Input: part model. Units: mm. Frame: model coordinates. A direction names the side the tool comes from. Coordinates: 2 decimals unless noted, no trailing zeros.
1) Section query A-A (z = 2). State how many separate pieces and enclosed holes the cut face has, then the cut area to 3 significant figures.
2) Set-up query: faces 1 (the flat face through (132, -3.5, 3)), 2 (the cylindrical face through (36.819, -50.474, 4.521)), 3 (the flat face through (122.848, -37.563, 2.958)), 4 (the flat face through (-135, -1, 3)), 5 (the flat face through (-75, 83, 3)). Return all of +Z, -Z, +X, -X, +Y, -Y with unobstructed straight access to the full face (end or side cutting, diameter ignored); none if empty.
3) Draft query along Y for faces 6 (the flat face through (-35, 106.5, 3)), 7 (the flat face through (-72, 75.5, 3)), 8 (the flat face through (65, 109, 3)), 9 (the flat face through (110.085, -35.626, 2.958)). Return one class per face: pulls with the +Y half, pulls with the -Y half, needs draft (parallel to the pull), parting line crosses it, or undercut.
4) Pin query (flat end, axial travel): pin 1 Ø3 at (y, z) = (37, 2.5) entering from +X; pin 2 Ø5 at (x, y) = (132, 9) entering from +Z; pin 3 Ø2 at (y, z) = (-85, 3.5) entering from +X. Return the tip coordinate at first contact, or that it passes through.
5) Line query: L1, parallel to Y at x = 102.5, z = 3.75; L2, parallel to X at y = 97.5, z = 2.4; L3, parallel to Y at x = -101.5, z = 2. Output: solid intervals per line, ascending.
from build123d import *

# Parameters (mm, degrees)
ESQUISSE1_W                   = 270
ESQUISSE1_H                   = 213
BOSS_EXTRU_1_DEPTH            = 6
ESQUISSE3_R                   = 9.45
ESQUISSE3_R_2                 = 1.5
ENL_V_MAT_EXTRU_1_DEPTH       = 10
ENL_V_MAT_EXTRU_11_DEPTH      = 173.055950202
ENL_V_MAT_EXTRU_11_DEPTH_BACK = 173.055950202
ESQUISSE7_W                   = 6
ESQUISSE7_H                   = 30
ESQUISSE7_H_2                 = 27
ENL_V_MAT_EXTRU_13_DEPTH      = 10
ESQUISSE8_W                   = 40
ESQUISSE8_H                   = 6
BOSS_EXTRU_2_DEPTH            = 6
ENL_V_MAT_EXTRU_14_DEPTH      = 10
ENL_V_MAT_EXTRU_15_DEPTH      = 6
ESQUISSE11_W                  = 6
ESQUISSE11_H                  = 15
ENL_V_MAT_EXTRU_16_DEPTH      = 10
ESQUISSE14_W                  = 30
ESQUISSE14_H                  = 6
BOSS_EXTRU_3_DEPTH            = 6
ENL_V_MAT_EXTRU_18_DEPTH      = 176.833017377
ESQUISSE17_R                  = 2.995
ESQUISSE17_R_2                = 3
ENL_V_MAT_EXTRU_20_DEPTH      = 3
ESQUISSE18_R                  = 1.5
ENL_V_MAT_EXTRU_21_DEPTH      = 13


with BuildPart() as part:
    # Esquisse1 → Boss.-Extru.1 (new body)
    with BuildSketch(Plane.XY):
        Rectangle(ESQUISSE1_W, ESQUISSE1_H)
    extrude(amount=BOSS_EXTRU_1_DEPTH)

    # Esquisse3 → Enlèv. mat.-Extru.1 (cut)
    with BuildSketch(Plane.XY.offset(6)):
        with Locations((-100, -21.5)):
            Circle(ESQUISSE3_R)
        with Locations((35.99, -3.47)):
            Circle(ESQUISSE3_R_2)
        with Locations((43.49, 9.52)):
            Circle(ESQUISSE3_R_2)
        with Locations((44.65, -8.50726277)):
            Circle(ESQUISSE3_R_2)
        with Locations((52.15, 4.48273723)):
            Circle(ESQUISSE3_R_2)
        with Locations((71.2, -6.51726277)):
            Circle(ESQUISSE3_R_2)
        with Locations((63.7, -19.50726277)):
            Circle(ESQUISSE3_R_2)
        with Locations((72.36, -24.962747355)):
            Circle(ESQUISSE3_R_2)
        with Locations((79.86, -11.972747355)):
            Circle(ESQUISSE3_R_2)
    extrude(amount=-ENL_V_MAT_EXTRU_1_DEPTH, mode=Mode.SUBTRACT)

    # Esquisse5 → Enlèv. mat.-Extru.11 (cut, two sides: drawn at the far end of the back side and taken through both)
    with BuildSketch(Plane.XY.offset(6).offset(-ENL_V_MAT_EXTRU_11_DEPTH_BACK)):
        Polygon((135, -36.5), (53.963742643, -43.589753853), (-55, -106.5), (135, -106.5), align=None)
    extrude(amount=ENL_V_MAT_EXTRU_11_DEPTH + ENL_V_MAT_EXTRU_11_DEPTH_BACK, mode=Mode.SUBTRACT)

    # Esquisse7 → Enlèv. mat.-Extru.13 (cut)
    with BuildSketch(Plane.XY.offset(6)):
        with Locations((132, 91.5)):
            Rectangle(ESQUISSE7_W, ESQUISSE7_H)
        with Locations((132, -17)):
            Rectangle(ESQUISSE7_W, ESQUISSE7_H_2)
        with Locations((132, 34)):
            Rectangle(ESQUISSE7_W, ESQUISSE7_H_2)
    extrude(amount=-ENL_V_MAT_EXTRU_13_DEPTH, mode=Mode.SUBTRACT)

    # Esquisse8 → Boss.-Extru.2 (add)
    with BuildSketch(Plane(origin=(0, 106.5, 0), x_dir=(1, 0, 0), z_dir=(0, 1, 0))):
        with Locations((85, -3)):
            Rectangle(ESQUISSE8_W, ESQUISSE8_H)
        with Locations((5, -3)):
            Rectangle(ESQUISSE8_W, ESQUISSE8_H)
        with Locations((-75, -3)):
            Rectangle(ESQUISSE8_W, ESQUISSE8_H)
    extrude(amount=BOSS_EXTRU_2_DEPTH)

    # Esquisse9 → Enlèv. mat.-Extru.14 (cut)
    with BuildSketch(Plane(origin=(0, 0, 0), x_dir=(-1, 0, 0), z_dir=(0, 0, -1))):
        Polygon((-110.35, -38.656595556), (-79.413742643, -41.363167367), (-78.890808186, -35.385999178), (-109.827065544, -32.679427367), align=None)
    extrude(amount=-ENL_V_MAT_EXTRU_14_DEPTH, mode=Mode.SUBTRACT)

    # Esquisse10 → Enlèv. mat.-Extru.15 (cut)
    with BuildSketch(Plane(origin=(0, 0, 0), x_dir=(-1, 0, 0), z_dir=(0, 0, -1))):
        Polygon((-32.03555308, -56.25), (-10.384917986, -68.75), (-7.384917986, -63.553847577), (-29.03555308, -51.053847577), align=None)
        Polygon((11.265717109, -81.25), (32.916352203, -93.75), (35.916352203, -88.553847577), (14.265717109, -76.053847577), align=None)
    extrude(amount=-ENL_V_MAT_EXTRU_15_DEPTH, mode=Mode.SUBTRACT)

    # Esquisse11 → Enlèv. mat.-Extru.16 (cut)
    with BuildSketch(Plane(origin=(0, 0, 0), x_dir=(-1, 0, 0), z_dir=(0, 0, -1))):
        with Locations((72, 52)):
            Rectangle(ESQUISSE11_W, ESQUISSE11_H)
        with Locations((72, 83)):
            Rectangle(ESQUISSE11_W, ESQUISSE11_H)
    extrude(amount=-ENL_V_MAT_EXTRU_16_DEPTH, mode=Mode.SUBTRACT)

    # Esquisse14 → Boss.-Extru.3 (add)
    with BuildSketch(Plane.XZ.offset(106.5)):
        with Locations((-95, 3)):
            Rectangle(ESQUISSE14_W, ESQUISSE14_H)
    extrude(amount=BOSS_EXTRU_3_DEPTH)

    # Esquisse15 → Enlèv. mat.-Extru.18 (cut, through all)
    with BuildSketch(Plane.XY.offset(6)):
        Polygon((105, 106.5), (129, 106.5), (129, 76.5), align=None)
    extrude(amount=-ENL_V_MAT_EXTRU_18_DEPTH, mode=Mode.SUBTRACT)

    # Esquisse17 → Enlèv. mat.-Extru.20 (cut)
    with BuildSketch(Plane.XY.offset(6)):
        with Locations((-75, 109.5)):
            Circle(ESQUISSE17_R)
        with Locations((5, 109.5)):
            Circle(ESQUISSE17_R)
        with Locations((85, 109.5)):
            Circle(ESQUISSE17_R)
        with Locations((132, 60)):
            Circle(ESQUISSE17_R)
        with Locations((132, 9)):
            Circle(ESQUISSE17_R)
        with Locations((-1.940399562, -72.401923789)):
            Circle(ESQUISSE17_R)
        with Locations((119.054285055, -34.883609777)):
            Circle(ESQUISSE17_R)
        with Locations((66.699841688, -39.464030057)):
            Circle(ESQUISSE17_R)
        with Locations((-45.241669751, -97.401923789)):
            Circle(ESQUISSE17_R)
        with Locations((-95, -109.5)):
            Circle(ESQUISSE17_R)
        with Locations((39.195807118, -48.651923789)):
            Circle(ESQUISSE17_R)
        with Locations((-72, 67.5)):
            Circle(ESQUISSE17_R_2)
        with Locations((-72, 37.5)):
            Circle(ESQUISSE17_R_2)
        with Locations((-72, 97.5)):
            Circle(ESQUISSE17_R)
    extrude(amount=-ENL_V_MAT_EXTRU_20_DEPTH, mode=Mode.SUBTRACT)

    # Esquisse18 → Enlèv. mat.-Extru.21 (cut)
    with BuildSketch(Plane.XY.offset(6)):
        with Locations((-75, 109.5)):
            Circle(ESQUISSE18_R)
        with Locations((5, 109.5)):
            Circle(ESQUISSE18_R)
        with Locations((85, 109.5)):
            Circle(ESQUISSE18_R)
        with Locations((132, 60)):
            Circle(ESQUISSE18_R)
        with Locations((132, 9)):
            Circle(ESQUISSE18_R)
        with Locations((119.054285055, -34.883609777)):
            Circle(ESQUISSE18_R)
        with Locations((66.699841688, -39.464030057)):
            Circle(ESQUISSE18_R)
        with Locations((-1.940399562, -72.401923789)):
            Circle(ESQUISSE18_R)
        with Locations((-45.241669751, -97.401923789)):
            Circle(ESQUISSE18_R)
        with Locations((-72, 97.5)):
            Circle(ESQUISSE18_R)
        with Locations((-72, 67.5)):
            Circle(ESQUISSE18_R)
        with Locations((-72, 37.5)):
            Circle(ESQUISSE18_R)
        with Locations((-95, -109.5)):
            Circle(ESQUISSE18_R)
        with Locations((39.195807118, -48.651923789)):
            Circle(ESQUISSE18_R)
        with Locations((-93, 102.5)):
            Circle(ESQUISSE18_R)
    extrude(amount=-ENL_V_MAT_EXTRU_21_DEPTH, mode=Mode.SUBTRACT)


solid = part.part
Answer:
1. separate pieces: 1
1. enclosed holes: 26
1. area: 47,600 mm2
2. face 1: +Z, -Z, +X
2. face 2: +Z
2. face 3: +Z, -Z, +X, -Y
2. face 4: +Z, -Z, -X, +Y, -Y
2. face 5: +Z, -Z
3. face 6: pulls with the +Y half
3. face 7: undercut
3. face 8: needs draft
3. face 9: pulls with the -Y half
4. pin 1: stops at x = 129
4. pin 2: stops at z = 3
4. pin 3: stops at x = -28.03
5. L1: y = -33.32 to 112.5
5. L2: x = -135 to -73.5, -70.5 to 112.2
5. L3: y = -112.5 to -30.83, -12.17 to 106.5
